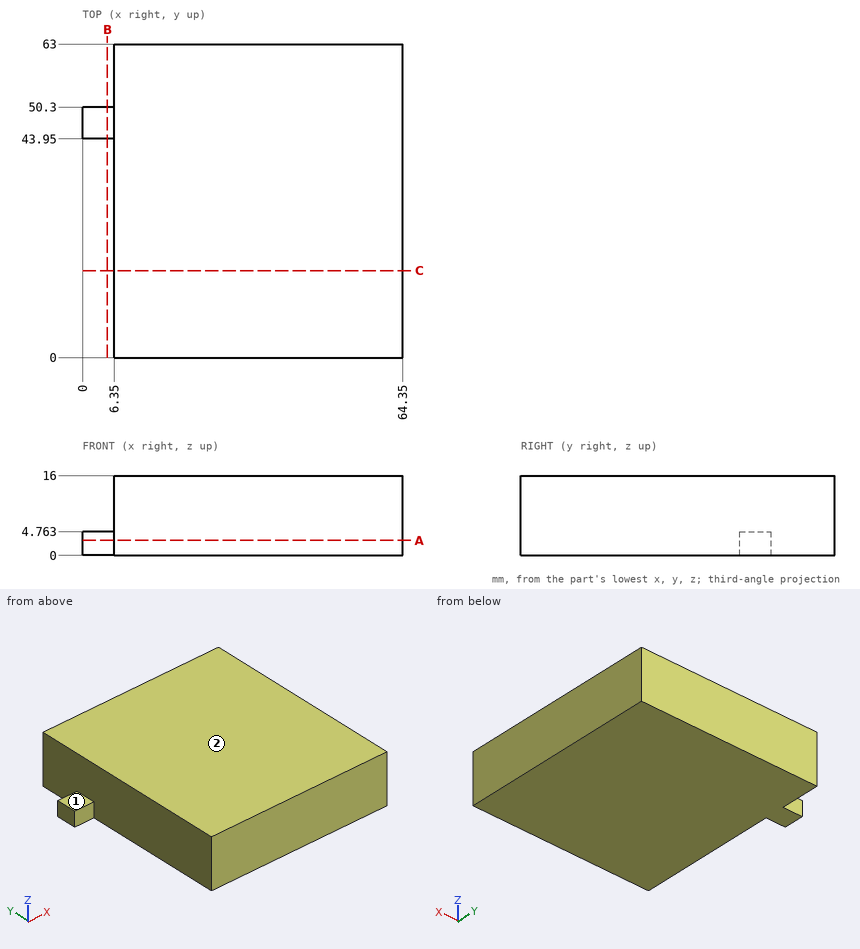
Input: dimensioned drawing with shaded views. Units: mm. Origin: part minimum x, y, z. A direction names the side the tool comes from. Round coordinates to 2 decimals unless told otherwise and drop trailing zeros. Loops run counter-clockwise (first coordinate to the right, second up) from the corner with the lowest first, then second, coordinate; pieces in that order, holes last. Notation, with made-up numbers: (-4.5, 19) -> (50.5, 19) arc R13 ccw to (50.5, 28) -> close; hole circle Ø5 at (74, 29). An arc over 180 degrees is marked (long way). Answer as a JSON object with one key per item and string values. Group by question number.
1) Section query B-B on x = 5. Output: boundary loops of the cut face in (y, z).
2) Ray query, L1, parallel to X at y = 15, z = 3.5. Return the intervals inside material, ascending.
3) Section query A-A on z = 3. Output: boundary loops of the cut face in (x, y).
4) Reachability of the marked faces 1 and 2 from +Z, -Z, +X, -X, +Y, -Y: full face, straight path, thin tool, end or side. Return the list, or none.
5) Pin query (flat end, axial travel): pin 1 (5 mm diameter, centred on y = 36, z = 2.5, fed in from -X); pin 2 (4 mm diameter, centred on x = 2.5, z = 1, fed in from -Y); pin 3 (3 mm diameter, centred on x = 4, y = 48.5, fed in from +Z). Return the tip coordinate at first contact, or that it passes through.
6) Section query C-C on y = 17.5. Output: boundary loops of the cut face in (x, z).
Reply:
{
 "1": {"outline": "(43.95, 0) -> (50.3, 0) -> (50.3, 4.76) -> (43.95, 4.76) -> close"},
 "2": {"L1": "x = 6.35 to 64.35"},
 "3": {"outline": "(0, 43.95) -> (6.35, 43.95) -> (6.35, 0) -> (64.35, 0) -> (64.35, 63) -> (6.35, 63) -> (6.35, 50.3) -> (0, 50.3) -> close"},
 "4": {"face 1": "+Z, -X, +Y, -Y", "face 2": "+Z, +X, -X, +Y, -Y"},
 "5": {"pin 1": "stops at x = 6.35", "pin 2": "stops at y = 43.95", "pin 3": "stops at z = 4.76"},
 "6": {"outline": "(6.35, 0) -> (64.35, 0) -> (64.35, 16) -> (6.35, 16) -> close"}
}
